Part model, mm, in its own coordinate system. Face numbers are marked on the shaded views. A direction names the side the tool comes from. Give positions to 0.01 mm unless a question says otherwise; leave off trailing zeros. Write each loop counter-clockwise with the first axis right and the second up, starting at its lowest first coordinate (ties: lowest second). Pieces come first, ordered by that corner, then holes.
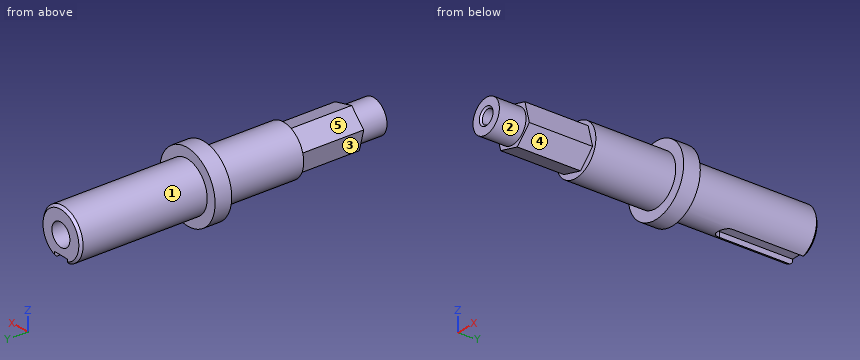
```python
from build123d import *

# Parameters (mm, degrees)
ESBO_O2_W                                      = 5
ESBO_O2_H                                      = 6
CORTE_EXTRUS_O1_DEPTH                          = 22
CORTE_EXTRUS_O2_DEPTH                          = 2
ESBO_O5_R                                      = 12.651043405
CORTE_EXTRUS_O8_DEPTH                          = 19
BROCA_DE_ROSQUEAR_PARA_TARRAXA_DE_M5X0_8_D     = 4.2
BROCA_DE_ROSQUEAR_PARA_TARRAXA_DE_M5X0_8_DEPTH = 10
BROCA_DE_ROSQUEAR_PARA_TARRAXA_DE_M5X0_8_TIP   = 1.2618073
CHANFRO1_SIZE                                  = 0.5
ESBO_O10_W                                     = 3
ESBO_O10_H                                     = 5
BROCA_DE_ROSQUEAR_PARA_TARRAXA_DE_M81_D        = 6.8
BROCA_DE_ROSQUEAR_PARA_TARRAXA_DE_M81_DEPTH    = 20
BROCA_DE_ROSQUEAR_PARA_TARRAXA_DE_M81_TIP      = 2.042926105


with BuildPart() as part:
    # Esboço1 → Revolução1 (revolve)
    with BuildSketch(Plane.XY, mode=Mode.PRIVATE) as revolu_o1_sk:
        Polygon((6.792893219, 47), (4, 47), (0, 47), (0, 23), (0, -47), (5, -47), (5, -39), (7.5, -39), (7.5, -11), (7.5, 46.292893219), align=None)
    revolve(revolu_o1_sk.sketch.rotate(Axis((0, -47, 0), (0, -1, 0)), 90), axis=Axis((0, -47, 0), (0, -1, 0)))

    # Esboço2 → Corte-extrusão1 (cut)
    with BuildSketch(Plane(origin=(0, 47, 0), x_dir=(1, 0, 0), z_dir=(0, 1, 0))):
        with Locations((0, 8.5)):
            Rectangle(ESBO_O2_W, ESBO_O2_H)
    extrude(amount=-CORTE_EXTRUS_O1_DEPTH, mode=Mode.SUBTRACT)

    # Esboço3 → Corte-extrusão2 (cut)
    with BuildSketch(Plane(origin=(0, 25, -7.5), x_dir=(-1, 0, 0), z_dir=(0, 0, -1))):
        with BuildLine():
            Line((2.5, 0), (-2.5, 0))
            ThreePointArc((-2.5, 0), (0, -2.5), (2.5, 0))
        make_face()
    extrude(amount=-CORTE_EXTRUS_O2_DEPTH, mode=Mode.SUBTRACT)

    # Esboço5 → Corte-extrusão8 (cut)
    with BuildSketch(Plane.XZ.offset(39)):
        Circle(ESBO_O5_R)
        Polygon((-4.596194078, -4.596194078), (1.682323793, -6.278517871), (6.278517871, -1.682323793), (4.596194078, 4.596194078), (-1.682323793, 6.278517871), (-6.278517871, 1.682323793), align=None, mode=Mode.SUBTRACT)
    extrude(amount=-CORTE_EXTRUS_O8_DEPTH, mode=Mode.SUBTRACT)

    # Broca de rosquear para tarraxa de M5x0.81
    with Locations(Plane(origin=(0, -47, 0), x_dir=(-1, 0, 0), z_dir=(0, -1, 0))):
        with Locations((0, 0)):
            Hole(BROCA_DE_ROSQUEAR_PARA_TARRAXA_DE_M5X0_8_D / 2, depth=BROCA_DE_ROSQUEAR_PARA_TARRAXA_DE_M5X0_8_DEPTH)
            with Locations((0, 0, -(BROCA_DE_ROSQUEAR_PARA_TARRAXA_DE_M5X0_8_DEPTH + BROCA_DE_ROSQUEAR_PARA_TARRAXA_DE_M5X0_8_TIP / 2))):  # 118° drill point
                Cone(0, BROCA_DE_ROSQUEAR_PARA_TARRAXA_DE_M5X0_8_D / 2, BROCA_DE_ROSQUEAR_PARA_TARRAXA_DE_M5X0_8_TIP, mode=Mode.SUBTRACT)

    # Chanfro1
    chanfro1_edges = [part.edges().sort_by_distance(p)[0] for p in [
        (-2.1, -47, 0),
    ]]
    chamfer(chanfro1_edges, length=CHANFRO1_SIZE)

    # Esboço10 → Revolução2 (revolve)
    with BuildSketch(Plane(origin=(0, 0, 0), x_dir=(-0.965925826289067, 0, 0.2588190451025257), z_dir=(-0.2588190451025257, 0, -0.965925826289067)), mode=Mode.PRIVATE) as revolu_o2_sk:
        with Locations((9, 6.5)):
            Rectangle(ESBO_O10_W, ESBO_O10_H)
    revolve(revolu_o2_sk.sketch.rotate(Axis((0, -20, 0), (0, 1, 0)), 165), axis=Axis((0, -20, 0), (0, 1, 0)))

    # Broca de rosquear para tarraxa de M81
    with Locations(Plane(origin=(0, 47, 0), x_dir=(1, 0, 0), z_dir=(0, 1, 0))):
        with Locations((0, 0)):
            Hole(BROCA_DE_ROSQUEAR_PARA_TARRAXA_DE_M81_D / 2, depth=BROCA_DE_ROSQUEAR_PARA_TARRAXA_DE_M81_DEPTH)
            with Locations((0, 0, -(BROCA_DE_ROSQUEAR_PARA_TARRAXA_DE_M81_DEPTH + BROCA_DE_ROSQUEAR_PARA_TARRAXA_DE_M81_TIP / 2))):  # 118° drill point
                Cone(0, BROCA_DE_ROSQUEAR_PARA_TARRAXA_DE_M81_D / 2, BROCA_DE_ROSQUEAR_PARA_TARRAXA_DE_M81_TIP, mode=Mode.SUBTRACT)


solid = part.part
```
1) Saw through at B-B, the plane y = 13.5. Write the cut outline in (x, z), then the cut area to 3 significant figures.
Answers follow:
outline: circle Ø15 at (0, 0)
area: 177 mm2
2) Wall check: L1, parallel to X at y = -43.5, z = 0; L2, parallel to Y at x = -0.75, z = 8; L3, parallel to Z at x = 0, y = 41.25. Give the ranges that are in metal, low to high.
Answers follow:
L1: x = -5 to -2.1, 2.1 to 5
L2: y = 4 to 9
L3: z = -5.5 to -3.4, 3.4 to 7.5
3) Pin check, flat tips, straight feed: pin 1 Ø0.5 at (y, z) = (33, -6) entering from -X; pin 2 Ø1.5 at (y, z) = (-21, -5) entering from -X; pin 3 Ø1 at (y, z) = (35.5, -2) entering from -X. Stop position of each tip, or through.
Answers follow:
pin 1: stops at x = -4.82
pin 2: stops at x = -4.69
pin 3: stops at x = -7.35
4) Saw through at A-A, the plane y = 28. Write the cut outline in (x, z), then the cut area to 3 significant figures.
Answers follow:
outline: (-2.5, -7.07) - (-2.5, -5.5) - (2.5, -5.5) - (2.5, -7.07) arc R7.5 ccw (long way) to start; hole circle Ø6.8 at (0, 0)
area: 131 mm2
5) 3-axis set-ups, long thin cutter, end or side, ignore diameter. For the marked faces 1, 2, 3, 4 and 5: which of +Z, -Z, +X, -X, +Y, -Y reach the whole face in a straight line?
Answers follow:
face 1: +Y
face 2: -Y
face 3: -Z, -X, -Y
face 4: -Z, +X, -Y
face 5: +Z, -X, -Y
